Design review of the part built by this model. Coordinates are the model's own, in mm. Give positions to 0.01 mm unless a question says otherwise; leave off trailing zeros. Loops run counter-clockwise (first coordinate to the right, second up) from the corner with the lowest first, then second, coordinate; pieces in that order, holes last. Notation, with made-up numbers: (28.25, 43) -> (85.25, 43) arc R19 ccw to (85.25, 73) -> close; hole circle Ø5 at (0, -35). An arc over 180 degrees is marked (long way). Use a Markdown table: item, result. Add a question column.
1. For pin 1 Ø4.5 at (x, y) = (12.7, 128.27) entering from +Z, flat-tipped, find the tip position at first contact; note if it passes through.
2. Draft analysis for pull direction Y (two halves, no side actions). For faces 1 (the cylindrical face through (24.636, 132.626, -0.373)), 2 (the cylindrical face through (13.19, 89.48, -0.37)), 3 (the flat face through (13, 68, 0)), state which applies: pulls with the +Y half, pulls with the -Y half, needs draft (parallel to the pull), parting line crosses it, or undercut.
3. Add section A-A (x = 12.7). State the section outline as (y, z) points (3 decimals), and give its area (3 significant figures).
4. Add section B-B (y = 5.08). State the section outline as (x, z) points, and give its area (3 significant figures).
5. To check wall thickness, follow line 1 (Y direction, x = 12.75, z = -0.05); line 2 (Y direction, x = 13, z = -0.55); line 3 (X direction, y = 128.27, z = -0.4). State the ranges of each line that lie inside material, in increasing order.
6. Add section C-C (z = -0.25). State the section outline as (x, y) points (3 decimals).
```python
from build123d import *

# Parameters (mm, degrees)
SKETCH1_W                       = 25.4
SKETCH1_H                       = 133.35
BASE_FLANGE1_DEPTH              = 0.7366
BREAK_CORNER1_START             = -0.7366
BREAK_CORNER1_DEPTH             = 0.7366
M4_CLEARANCE_HOLE2_D            = 4.5
F_5_32_0_15625_DIAMETER_HOLE2_D = 3.96875


# Read off the part's stored shape, not the designer's step: Break-Corner1
# Sheet-metal steps are written as plain solids
with BuildPart() as part:
    # Sketch1 → Base-Flange1 (new body)
    with BuildSketch(Plane.XY):
        with Locations((12.7, 66.675)):
            Rectangle(SKETCH1_W, SKETCH1_H)
    extrude(amount=-BASE_FLANGE1_DEPTH)

    # Break-Corner1 outline → Break-Corner1 (cut)
    with BuildSketch(Plane.XY.offset(BREAK_CORNER1_START)):
        with BuildLine():
            ThreePointArc((2.54, 0), (0.743948776, 0.743948776), (0, 2.54))
            Line((0, 2.54), (0, 0))
            Line((0, 0), (2.54, 0))
        make_face()
        with BuildLine():
            Line((0, 133.35), (0, 130.81))
            ThreePointArc((0, 130.81), (0.743948776, 132.606051224), (2.54, 133.35))
            Line((2.54, 133.35), (0, 133.35))
        make_face()
        with BuildLine():
            ThreePointArc((25.4, 2.54), (24.656051224, 0.743948776), (22.86, 0))
            Line((22.86, 0), (25.4, 0))
            Line((25.4, 0), (25.4, 2.54))
        make_face()
        with BuildLine():
            Line((25.4, 133.35), (22.86, 133.35))
            ThreePointArc((22.86, 133.35), (24.656051224, 132.606051224), (25.4, 130.81))
            Line((25.4, 130.81), (25.4, 133.35))
        make_face()
    extrude(amount=BREAK_CORNER1_DEPTH, mode=Mode.SUBTRACT)

    # M4 Clearance Hole2 (through all)
    with Locations(Plane.XY):
        with Locations((12.7, 91.675), (12.7, 41.675)):
            Hole(M4_CLEARANCE_HOLE2_D / 2)

    # 5/32 (0.15625) Diameter Hole2 (through all)
    with Locations(Plane.XY):
        with Locations((12.7, 5.08), (12.7, 128.27)):
            Hole(F_5_32_0_15625_DIAMETER_HOLE2_D / 2)


solid = part.part
```
Taken from the geometry:
| question | item | result |
|---|---|---|
| 1 | pin 1 | stops at z = 0 |
| 2 | face 1 | pulls with the +Y half |
| 2 | face 2 | undercut |
| 2 | face 3 | needs draft |
| 3 | outline | (0, -0.737) -> (3.096, -0.737) -> (3.096, 0) -> (0, 0) -> close; (7.064, -0.737) -> (39.425, -0.737) -> (39.425, 0) -> (7.064, 0) -> close; (43.925, -0.737) -> (89.425, -0.737) -> (89.425, 0) -> (43.925, 0) -> close; (93.925, -0.737) -> (126.286, -0.737) -> (126.286, 0) -> (93.925, 0) -> close; (130.254, -0.737) -> (133.35, -0.737) -> (133.35, 0) -> (130.254, 0) -> close |
| 3 | area | 85.7 mm^2 |
| 4 | outline | (0, -0.74) -> (10.72, -0.74) -> (10.72, 0) -> (0, 0) -> close; (14.68, -0.74) -> (25.4, -0.74) -> (25.4, 0) -> (14.68, 0) -> close |
| 4 | area | 15.8 mm^2 |
| 5 | line 1 | y = 0 to 3.1, 7.06 to 39.43, 43.92 to 89.43, 93.92 to 126.29, 130.25 to 133.35 |
| 5 | line 2 | y = 0 to 3.12, 7.04 to 39.45, 43.9 to 89.45, 93.9 to 126.31, 130.23 to 133.35 |
| 5 | line 3 | x = 0 to 10.72, 14.68 to 25.4 |
| 6 | outline | (0, 2.54) arc R2.54 ccw to (2.54, 0) -> (22.86, 0) arc R2.54 ccw to (25.4, 2.54) -> (25.4, 130.81) arc R2.54 ccw to (22.86, 133.35) -> (2.54, 133.35) arc R2.54 ccw to (0, 130.81) -> close; hole circle Ø4.5 at (12.7, 41.675); hole circle Ø4.5 at (12.7, 91.675); hole circle Ø3.969 at (12.7, 5.08); hole circle Ø3.969 at (12.7, 128.27) |
